Can you work these out from the model? Positions are in its coordinate system, mm. Round coordinates to 2 decimals unless told otherwise and drop trailing zeros. Order: outer loops, then holes, each group sorted by start corner. A loop starts at its lowest first (then second) coordinate and runs counter-clockwise, first axis right, second up. Notation, with made-up numbers: M 33,89 L 89,89 A32 cw 89,120 Z; hole C -13,15 d6. An arc over 180 degrees is marked long. Answer as a JSON object with one key per item and string values. Group by question number.
```python
from build123d import *

# Parameters (mm, degrees)
SKETCH1_R           = 1.3462
SKETCH1_W           = 3.7846
SKETCH1_H           = 52.6961
BOSS_EXTRUDE1_DEPTH = 3.048
SKETCH2_R           = 1.524
CUT_EXTRUDE1_DEPTH  = 4.048
CUT_EXTRUDE2_DEPTH  = 4.048


with BuildPart() as part:
    # Sketch1 → Boss-Extrude1 (new body)
    with BuildSketch(Plane.XY):
        with BuildLine():
            Line((-401.0571, 150.956597849), (-401.0571, 148.341))
            Line((-401.0571, 148.341), (-399.1521, 148.341))
            Line((-399.1521, 148.341), (-395.3675, 148.341))
            Line((-395.3675, 148.341), (-395.3675, 149.2432))
            Line((-395.3675, 149.2432), (-309.8086, 149.2432))
            Line((-309.8086, 149.2432), (-309.8086, 128.8851))
            Line((-309.8086, 128.8851), (-305.87795, 128.8851))
            Line((-305.87795, 128.8851), (-301.9473, 132.81575))
            Line((-301.9473, 132.81575), (-301.9473, 150.9704))
            ThreePointArc((-301.9473, 150.9704), (-303.063223164, 153.664476836), (-305.7573, 154.7804))
            Line((-305.7573, 154.7804), (-397.247125, 154.7804))
            ThreePointArc((-397.247125, 154.7804), (-399.946077222, 153.659592612), (-401.0571, 150.956597849))
        make_face()
        with Locations((-397.247125, 150.9704)):
            Circle(SKETCH1_R, mode=Mode.SUBTRACT)
        with Locations((-305.7573, 150.9704)):
            Circle(SKETCH1_R, mode=Mode.SUBTRACT)
        with Locations((-397.2598, 121.99295)):
            Rectangle(SKETCH1_W, SKETCH1_H)
        with BuildLine():
            Line((-395.3675, 95.6449), (-399.1521, 95.6449))
            Line((-399.1521, 95.6449), (-401.0571, 95.6449))
            Line((-401.0571, 95.6449), (-401.0571, 91.659304166))
            ThreePointArc((-401.0571, 91.659304166), (-399.951018769, 88.947400452), (-397.2472, 87.8217))
            Line((-397.2472, 87.8217), (-378.5565, 87.8217))
            Line((-378.5565, 87.8217), (-368.3165, 91.1883))
            Line((-368.3165, 91.1883), (-315.9973, 91.1883))
            Line((-315.9973, 91.1883), (-305.7573, 87.8217))
            ThreePointArc((-305.7573, 87.8217), (-303.063223164, 88.937623164), (-301.9473, 91.6317))
            Line((-301.9473, 91.6317), (-301.9473, 111.74645))
            Line((-301.9473, 111.74645), (-305.87795, 115.6771))
            Line((-305.87795, 115.6771), (-309.8086, 115.6771))
            Line((-309.8086, 115.6771), (-309.8086, 92.9525))
            Line((-309.8086, 92.9525), (-395.3675, 92.9525))
            Line((-395.3675, 92.9525), (-395.3675, 95.6449))
        make_face()
        with Locations((-397.2472, 91.6317)):
            Circle(SKETCH1_R, mode=Mode.SUBTRACT)
        with Locations((-305.7573, 91.6317)):
            Circle(SKETCH1_R, mode=Mode.SUBTRACT)
    extrude(amount=BOSS_EXTRUDE1_DEPTH)

    # Sketch2 → Cut-Extrude1 (cut, through all)
    with BuildSketch(Plane(origin=(0, 0, 0), x_dir=(-1, 0, 0), z_dir=(0, 0, -1))):
        with Locations((305.7573, 150.9704)):
            Circle(SKETCH2_R)
        with Locations((305.7573, 91.6317)):
            Circle(SKETCH2_R)
        with Locations((397.2472, 91.6317)):
            Circle(SKETCH2_R)
        with Locations((397.247125, 150.9704)):
            Circle(SKETCH2_R)
    extrude(amount=-CUT_EXTRUDE1_DEPTH, mode=Mode.SUBTRACT)

    # Sketch3 → Cut-Extrude2 (cut, through all)
    with BuildSketch(Plane.XY.offset(3.048)):
        Polygon((-309.8086, 129.6471), (-309.8086, 128.8851), (-305.87795, 128.8851), (-301.9473, 132.81575), (-301.9473, 133.57775), (-305.87795, 129.6471), align=None)
        Polygon((-305.87795, 115.6771), (-309.8086, 115.6771), (-309.8086, 113.6451), (-305.87795, 113.6451), (-301.9473, 109.71445), (-301.9473, 111.74645), align=None)
    extrude(amount=-CUT_EXTRUDE2_DEPTH, mode=Mode.SUBTRACT)


solid = part.part
```
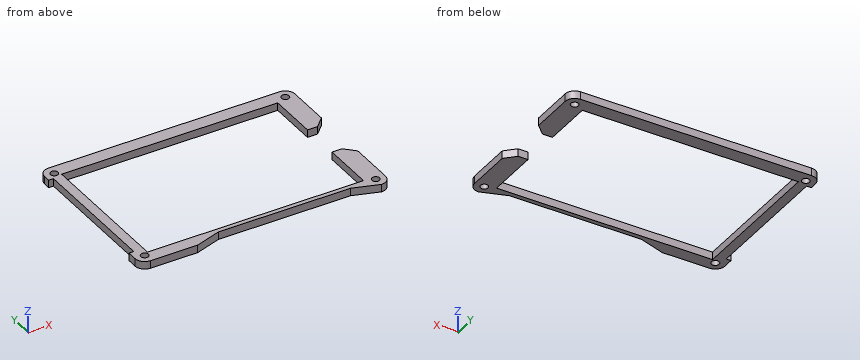
1) I need wall thicknesses on line 1 along X through (y, z) = (96.5, 2.95); line 2 along Y through (x, z) = (-322.5, 0.6); line 3 along Y through (x, z) = (-383, 1). Which ranges of each line are inside material? Lowest first, please.
2) For pin 1 (0.9 mm diameter, centred on x = -308, z = 1, fed in from -Y); pin 2 (1.5 mm diameter, centred on y = 121.5, z = 1.5, fed in from -X), each with a flat end and sliding along its axis, tell me the tip position at first contact or that it passes through.
3) If we section it at B-B on y = 136: Write out the boundary of the cut face in (x, z).
4) If we section it at A-A on x = -381: Write out the boundary of the cut face in (y, z), plus the area to 3 significant figures.
5) If we section it at C-C on z = 2: Count the separate pieces of the cut face and the enclosed holes in it, plus the area to 3 significant figures.
Findings:
{
 "1": {"line 1": "x = -399.15 to -395.37, -309.81 to -301.95", "line 2": "y = 91.19 to 92.95, 149.24 to 154.78", "line 3": "y = 87.82 to 92.95, 149.24 to 154.78"},
 "2": {"pin 1": "stops at y = 88.41", "pin 2": "stops at x = -399.15"},
 "3": {"outline": "M -399.15,0 L -395.37,0 L -395.37,3.05 L -399.15,3.05 Z; M -309.81,0 L -301.95,0 L -301.95,3.05 L -309.81,3.05 Z"},
 "4": {"outline": "M 87.82,0 L 92.95,0 L 92.95,3.05 L 87.82,3.05 Z; M 149.24,0 L 154.78,0 L 154.78,3.05 L 149.24,3.05 Z", "area": "32.5 mm^2"},
 "5": {"separate pieces": "1", "enclosed holes": "4", "area": "1,330 mm^2"}
}
